For this review, take the finished solid that the model builds, in its own axes (mm). Face numbers are marked on the shaded views. A direction names the side the tool comes from. Give positions to 0.01 mm unless a question says otherwise; leave off trailing zeros. Write each loop counter-clockwise with the first axis right and the second up, starting at its lowest first coordinate (ties: lowest second). Pieces come first, ordered by that corner, then holes.
1) We need section C-C on y = 6. Give the boundary of the cut face in (x, z), and give its area (3 significant figures).
2) Machinability: for the marked faces 1 and 2, which of the approach directions +Z, -Z, +X, -X, +Y, -Y give a long, thin tool a straight path to every point of the face, cutting with its end or side? Answer none if there is none.
3) We need section D-D on x = -14.25. Give the boundary of the cut face in (y, z), and give its area (3 significant figures).
4) Wall thickness on line 1 along Y through (x, z) = (-16.25, 7.75); line 2 along Y through (x, z) = (-17, 0.5); line 3 along X through (y, z) = (2.5, 5.75): over which ranges is each line inside the solid? List them lowest first.
5) We need section B-B on x = -16.5. Give the boundary of the cut face in (y, z).
6) We need section A-A on z = 5.5. Give the boundary of the cut face in (x, y), and give its area (3 significant figures).
7) For P1, Ø2.5, axis at x = -14, y = 2.5, coming from the +Z side; P2, Ø3.5, axis at x = -15.78, y = 1.96, coming from the +Z side, all flat-tipped, find the tip position at first contact; note any pin that passes through.
8) Draft analysis for pull direction X (two halves, no side actions). For the marked faces 3, 4, 5 and 6, state which applies: pulls with the +X half, pulls with the -X half, needs draft (parallel to the pull), parting line crosses it, or undercut.
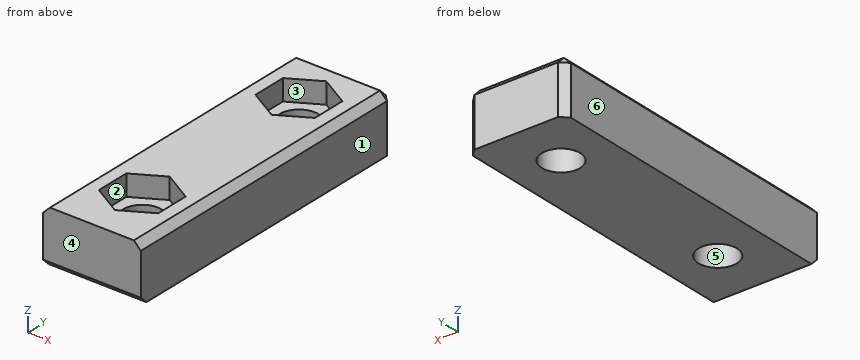
from build123d import *

# Parameters (mm, degrees)
F0_W     = 14
F0_H     = 45
F0_R     = 2.75
F1_DEPTH = 8
F3_DEPTH = 3
F4_SIZE  = 1


with BuildPart() as f1:
    # F0 (on Top) → F1 (new body)
    with BuildSketch(Plane.XY):
        with Locations((-15.778726, 15.456292)):
            Rectangle(F0_W, F0_H)
        with Locations((-15.778726, 1.956292)):
            Circle(F0_R, mode=Mode.SUBTRACT)
        with Locations((-15.778726, 29.956292)):
            Circle(F0_R, mode=Mode.SUBTRACT)
    extrude(amount=F1_DEPTH)

    # F2 (on face) → F3 (cut)
    with BuildSketch(Plane.XY.offset(8)):
        Polygon((-11.528726, 27.502553), (-11.528726, 32.41003), (-15.778726, 34.863769), (-20.028726, 32.41003), (-20.028726, 27.502553), (-15.778726, 25.048814), align=None)
        Polygon((-11.528726, -0.497447), (-11.528726, 4.41003), (-15.778726, 6.863769), (-20.028726, 4.41003), (-20.028726, -0.497447), (-15.778726, -2.951186), align=None)
    extrude(amount=-F3_DEPTH, mode=Mode.SUBTRACT)

    # F4
    f4_edges = [f1.edges().sort_by_distance(p)[0] for p in [
        (-15.778726, 37.956292, 8),
        (-8.778726, 37.956292, 4),
        (-22.778726, 37.956292, 4),
        (-15.778726, -7.043708, 0),
        (-8.778726, 15.456292, 8),
        (-22.778726, 15.456292, 8),
    ]]
    chamfer(f4_edges, length=F4_SIZE)


solid = f1.part
Results list:
1. outline: (-22.78, 0) - (-8.78, 0) - (-8.78, 7) - (-9.78, 8) - (-14.28, 8) - (-14.28, 5) - (-17.27, 5) - (-17.27, 8) - (-21.78, 8) - (-22.78, 7) - close
1. area: 102 mm2
2. face 1: +Z, -Z, +X, +Y, -Y
2. face 2: +Z
3. outline: (-7.04, 1) - (-6.04, 0) - (-0.33, 0) - (-0.33, 5) - (-2.07, 5) - (-2.07, 8) - (-7.04, 8) - close; (4.24, 0) - (27.67, 0) - (27.67, 5) - (25.93, 5) - (25.93, 8) - (5.98, 8) - (5.98, 5) - (4.24, 5) - close; (32.24, 0) - (37.96, 0) - (37.96, 7) - (36.96, 8) - (33.98, 8) - (33.98, 5) - (32.24, 5) - close
3. area: 265 mm2
4. line 1: y = -7.04 to -2.68, 6.59 to 25.32, 34.59 to 37.21
4. line 2: y = -6.54 to -0.51, 4.42 to 27.49, 32.42 to 37.96
4. line 3: x = -22.78 to -20.03, -11.53 to -8.78
5. outline: (-7.04, 1) - (-6.04, 0) - (-0.7, 0) - (-0.7, 5) - (-2.53, 5) - (-2.53, 8) - (-7.04, 8) - close; (4.61, 0) - (27.3, 0) - (27.3, 5) - (25.47, 5) - (25.47, 8) - (6.45, 8) - (6.45, 5) - (4.61, 5) - close; (32.61, 0) - (37.96, 0) - (37.96, 7) - (36.96, 8) - (34.45, 8) - (34.45, 5) - (32.61, 5) - close
6. outline: (-22.78, -7.04) - (-8.78, -7.04) - (-8.78, 36.96) - (-9.78, 37.96) - (-21.78, 37.96) - (-22.78, 36.96) - close; hole (-20.03, -0.5) - (-15.78, -2.95) - (-11.53, -0.5) - (-11.53, 4.41) - (-15.78, 6.86) - (-20.03, 4.41) - close; hole (-20.03, 27.5) - (-15.78, 25.05) - (-11.53, 27.5) - (-11.53, 32.41) - (-15.78, 34.86) - (-20.03, 32.41) - close
6. area: 504 mm2
7. P1: stops at z = 5
7. P2: passes through
8. face 3: undercut
8. face 4: needs draft
8. face 5: undercut
8. face 6: pulls with the -X half
